Build history of the part. All positions in model axes, mm. A direction names the side the tool comes from. Round coordinates to 2 decimals unless told otherwise and drop trailing zeros. Loops run counter-clockwise (first coordinate to the right, second up) from the corner with the lowest first, then second, coordinate; pieces in that order, holes last. Notation, with made-up numbers: (51, 58.25) - (103, 58.25) arc R28 cw to (103, 76.25) - close; hole circle Ø4 at (19.5, -13.75). An arc over 180 degrees is marked (long way). One line per question, with ' | ' between items. Start each with the question number.
from build123d import *

# Parameters (mm, degrees)
SKETCH_1_W          = 220
SKETCH_1_H          = 220
EXTRUDE_1_DEPTH     = 20
EXTRUDE_3_DEPTH     = 110
SKETCH_4_R          = 7.5
CUT_EXTRUDE_2_DEPTH = 5
SKETCH_7_R          = 7.5
CUT_EXTRUDE_3_DEPTH = 5
SKETCH_10_W         = 40
SKETCH_10_H         = 170
EXTRUDE_5_DEPTH     = 10
SKETCH_11_W         = 170
SKETCH_11_H         = 40
EXTRUDE_6_DEPTH     = 10
SKETCH_12_W         = 40
SKETCH_12_H         = 170
EXTRUDE_7_DEPTH     = 10
SKETCH_13_W         = 170
SKETCH_13_H         = 40
EXTRUDE_8_DEPTH     = 10
SKETCH_16_R         = 20
CUT_EXTRUDE_6_DEPTH = 20


# Read off the part's stored shape, not the designer's step: 镜向2, 镜向5
with BuildPart() as part:
    # 草图1 → 凸台-拉伸1 (new body)
    with BuildSketch(Plane.XY):
        Rectangle(SKETCH_1_W, SKETCH_1_H)
    extrude(amount=EXTRUDE_1_DEPTH)

    # 草图2 → 凸台-拉伸3 (add)
    with BuildSketch(Plane.XY.offset(20)):
        Polygon((85, 110), (110, 110), (110, 85), (90, 85), (90, 90), (85, 90), align=None)
    extrude(amount=EXTRUDE_3_DEPTH)

    # 草图4 → 切除-拉伸2 (cut)
    with BuildSketch(Plane(origin=(0, 85, 0), x_dir=(-1, 0, 0), z_dir=(0, -1, 0))):
        with Locations(Location((-100, -115, 0), (0, 0, 90))):
            Circle(SKETCH_4_R)
    extrude(amount=-CUT_EXTRUDE_2_DEPTH, mode=Mode.SUBTRACT)

    # 草图7 → 切除-拉伸3 (cut)
    with BuildSketch(Plane.ZY.offset(-85)):
        with Locations((115, 100)):
            Circle(SKETCH_7_R)
    extrude(amount=-CUT_EXTRUDE_3_DEPTH, mode=Mode.SUBTRACT)

    # 镜向2: part across plane


with BuildPart() as part_1:
    add(part.part)
    add(part.part.mirror(Plane(origin=(0, 0, 0), x_dir=(0, 0, 1), z_dir=(1, 0, 0))))

    # 镜向5: part across plane


with BuildPart() as part_2:
    add(part_1.part)
    add(part_1.part.mirror(Plane.ZX))

    # 草图10 → 凸台-拉伸5 (add)
    with BuildSketch(Plane(origin=(110, 0, 0), x_dir=(0, 0, -1), z_dir=(1, 0, 0))):
        with Locations((-40, 0)):
            Rectangle(SKETCH_10_W, SKETCH_10_H)
    extrude(amount=-EXTRUDE_5_DEPTH)

    # 草图11 → 凸台-拉伸6 (add)
    with BuildSketch(Plane.XZ.offset(110)):
        with Locations((0, 40)):
            Rectangle(SKETCH_11_W, SKETCH_11_H)
    extrude(amount=-EXTRUDE_6_DEPTH)

    # 草图12 → 凸台-拉伸7 (add)
    with BuildSketch(Plane.ZY.offset(110)):
        with Locations((40, 0)):
            Rectangle(SKETCH_12_W, SKETCH_12_H)
    extrude(amount=-EXTRUDE_7_DEPTH)

    # 草图13 → 凸台-拉伸8 (add)
    with BuildSketch(Plane(origin=(0, 110, 0), x_dir=(1, 0, 0), z_dir=(0, 1, 0))):
        with Locations((0, -40)):
            Rectangle(SKETCH_13_W, SKETCH_13_H)
    extrude(amount=-EXTRUDE_8_DEPTH)

    # 草图16 → 切除-拉伸6 (cut)
    with BuildSketch(Plane.XY.offset(20)):
        Circle(SKETCH_16_R)
    extrude(amount=-CUT_EXTRUDE_6_DEPTH, mode=Mode.SUBTRACT)


solid = part_2.part
1) Tool access for faces 1 (the flat face through (-1, 105, 60)), 2 (the flat face through (100, -90, 115)), 3 (the flat face through (-105, -1, 60)), 4 (the flat face through (100, -85, 74)): list every direction of +Z, -Z, +X, -X, +Y, -Y with a clear straight run to the whole face (end or side of a thin tool).
2) Two-plate mould, pull along Y, no slides. Class faces 5 (the flat face through (-110, 2, 35)), 6 (the flat face through (-2, 110, 35)), 7 (the flat face through (105, -1, 60)), 8 (the flat face through (-2, -110, 37)): +Y half, -Y half, draft (parallel to the pull), parting line (faces both ways), or undercut.
3) Saw through at B-B on z = 104.5. Write the cut outline in (x, y), and give its area (3 significant figures).
4) Drop flat-ended pins along their axis: pin 1 (8 mm diameter, centred on x = 2, y = -14, fed in from -Z); pin 2 (5 mm diameter, centred on x = 38.5, y = -107, fed in from +Z). Give the stop position or say it passes through.
5) Wall check: line 1 (Y direction, x = 87, z = 115); line 2 (Y direction, x = 0, z = 6); line 3 (Y direction, x = 85.5, z = 42). Give the ranges that are in metal, low to high. Write a range as [from, to].
6) Saw through at A-A on y = 0. Write the cut outline in (x, z).
7) Saw through at D-D on z = 43.5. Write the cut outline in (x, y).
Answer key:
1) face 1: +Z, +Y, -Y | face 2: none | face 3: +Z, +X, -X | face 4: +Z
2) face 5: draft | face 6: +Y half | face 7: undercut | face 8: -Y half
3) outline: (-110, -110) - (-85, -110) - (-85, -90) - (-90, -90) - (-90, -85) - (-110, -85) - close; (-110, 85) - (-90, 85) - (-90, 90) - (-85, 90) - (-85, 110) - (-110, 110) - close; (85, -110) - (110, -110) - (110, -85) - (90, -85) - (90, -90) - (85, -90) - close; (85, 90) - (90, 90) - (90, 85) - (110, 85) - (110, 110) - (85, 110) - close | area: 2,400 mm²
4) pin 1: through | pin 2: z = 60
5) line 1: [-110, -107.5], [-92.5, -90], [90, 92.5], [107.5, 110] | line 2: [-110, -20], [20, 110] | line 3: [-110, -90], [90, 110]
6) outline: (-110, 0) - (-20, 0) - (-20, 20) - (-100, 20) - (-100, 60) - (-110, 60) - close; (20, 0) - (110, 0) - (110, 60) - (100, 60) - (100, 20) - (20, 20) - close
7) outline: (-110, -110) - (110, -110) - (110, 110) - (-110, 110) - close; hole (-100, -85) - (-90, -85) - (-90, -90) - (-85, -90) - (-85, -100) - (85, -100) - (85, -90) - (90, -90) - (90, -85) - (100, -85) - (100, 85) - (90, 85) - (90, 90) - (85, 90) - (85, 100) - (-85, 100) - (-85, 90) - (-90, 90) - (-90, 85) - (-100, 85) - close
